Work out the finished part from the listing and answer in its coordinate system (mm). Face numbers are marked on the shaded views. Round coordinates to 2 decimals unless told otherwise and drop trailing zeros. Order: outer loops, then holes, each group sorted by start corner. A loop starts at its lowest first (then second) coordinate and runs counter-clockwise, first axis right, second up.
from build123d import *

# Parameters (mm, degrees)
SKETCH_1_W          = 30
SKETCH_1_H          = 20
EXTRUDE_1_DEPTH     = 2
SKETCH_2_R          = 1.25
CUT_EXTRUDE_1_DEPTH = 2
FILLET_1_R          = 2


with BuildPart() as part:
    # 草图1 → 凸台-拉伸1 (new body)
    with BuildSketch(Plane.XY):
        Rectangle(SKETCH_1_W, SKETCH_1_H)
    extrude(amount=EXTRUDE_1_DEPTH)

    # 草图2 → 切除-拉伸1 (cut)
    with BuildSketch(Plane.XY.offset(2)):
        with Locations((-10, -6.85)):
            Circle(SKETCH_2_R)
        with Locations((10, -6.85)):
            Circle(SKETCH_2_R)
    extrude(amount=-CUT_EXTRUDE_1_DEPTH, mode=Mode.SUBTRACT)

    # 圆角1
    fillet_1_edges = [part.edges().sort_by_distance(p)[0] for p in [
        (15, -10, 1),
        (-15, -10, 1),
        (-15, 10, 1),
        (15, 10, 1),
    ]]
    fillet(fillet_1_edges, radius=FILLET_1_R)


solid = part.part
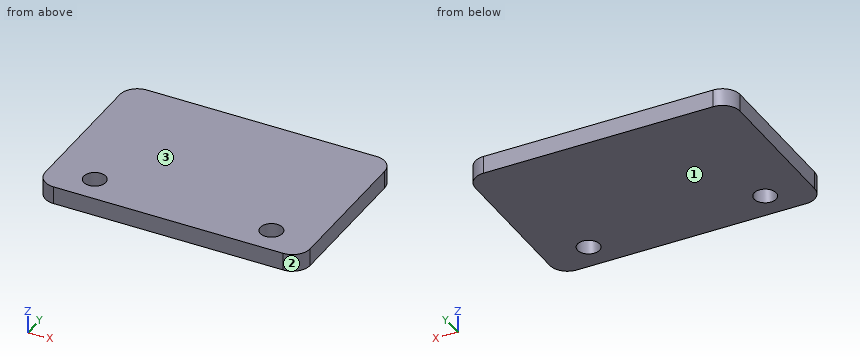
Item 1: Find section C-C (x = 10). Write down the section's boundary in (y, z), plus the area to 3 significant figures.
Item 2: Find the intervals of material crossed by line 1 along Y through (x, z) = (10, 1.3); line 2 along X through (y, z) = (-7.5, 0.1); line 3 along Y through (x, z) = (9.25, 0.35), in increasing order.
Item 3: Find section B-B (y = -6.85). Write down the section's boundary in (x, z).
Item 4: For a pull along Z with two mould halves and no side action, classify the marked faces 1, 2 and 3 as released by +Z, released by -Z, zero draft, split by the parting line, or undercut.
Item 5: Given pin 1 (1.5 mm diameter, centred on x = -10, y = -6.85, fed in from -Z); pin 2 (8 mm diameter, centred on x = 2, y = 1.5, fed in from -Z), each flat-ended and moving along its own axis, determine where each tip first touches the part or whether it passes through.
Item 6: Find section A-A (z = 0.7). Write down the section's boundary in (x, y), plus the area to 3 significant figures.
Model answer:
1. outline: (-10, 0) - (-8.1, 0) - (-8.1, 2) - (-10, 2) - close; (-5.6, 0) - (10, 0) - (10, 2) - (-5.6, 2) - close
1. area: 35.0 mm2
2. line 1: y = -10 to -8.1, -5.6 to 10
2. line 2: x = -15 to -11.07, -8.93 to 8.93, 11.07 to 15
2. line 3: y = -10 to -7.85, -5.85 to 10
3. outline: (-15, 0) - (-11.25, 0) - (-11.25, 2) - (-15, 2) - close; (-8.75, 0) - (8.75, 0) - (8.75, 2) - (-8.75, 2) - close; (11.25, 0) - (15, 0) - (15, 2) - (11.25, 2) - close
4. face 1: released by -Z
4. face 2: zero draft
4. face 3: released by +Z
5. pin 1: passes through
5. pin 2: stops at z = 0
6. outline: (-15, -8) arc R2 ccw to (-13, -10) - (13, -10) arc R2 ccw to (15, -8) - (15, 8) arc R2 ccw to (13, 10) - (-13, 10) arc R2 ccw to (-15, 8) - close; hole circle Ø2.5 at (-10, -6.85); hole circle Ø2.5 at (10, -6.85)
6. area: 587 mm2
